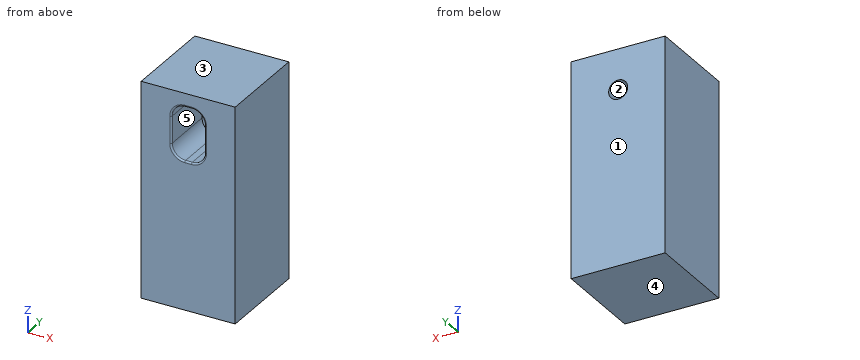
```python
from build123d import *

# Parameters (mm, degrees)
SKETCH1_W             = 22.225
SKETCH1_H             = 22.225
BOSS_EXTRUDE1_DEPTH   = 50.8
CUT_EXTRUDE1_DEPTH    = 12.7
F_8_CLEARANCE_HOLE1_D = 4.4958
FILLET1_R             = 0.381


with BuildPart() as part:
    # Sketch1 → Boss-Extrude1 (new body)
    with BuildSketch(Plane.XY):
        Rectangle(SKETCH1_W, SKETCH1_H)
    extrude(amount=BOSS_EXTRUDE1_DEPTH)

    # Sketch2 → Cut-Extrude1 (cut)
    with BuildSketch(Plane.XZ.offset(11.1125)):
        with BuildLine():
            Line((-0.79375, 47.625), (0.79375, 47.625))
            ThreePointArc((0.79375, 47.625), (3.03881403, 46.69506403), (3.96875, 44.45))
            Line((3.96875, 44.45), (3.96875, 38.1))
            ThreePointArc((3.96875, 38.1), (3.03881403, 35.85493597), (0.79375, 34.925))
            Line((0.79375, 34.925), (-0.79375, 34.925))
            ThreePointArc((-0.79375, 34.925), (-3.03881403, 35.85493597), (-3.96875, 38.1))
            Line((-3.96875, 38.1), (-3.96875, 44.45))
            ThreePointArc((-3.96875, 44.45), (-3.03881403, 46.69506403), (-0.79375, 47.625))
        make_face()
    extrude(amount=-CUT_EXTRUDE1_DEPTH, mode=Mode.SUBTRACT)

    # #8 Clearance Hole1 (through all)
    with Locations(Plane(origin=(0, 1.5875, 0), x_dir=(-1, 0, 0), z_dir=(0, -1, 0))):
        with Locations((0, -41.275)):
            Hole(F_8_CLEARANCE_HOLE1_D / 2)

    # Fillet1
    fillet1_edges = [part.edges().sort_by_distance(p)[0] for p in [
        (0, -11.1125, 47.625),
        (3.96875, -11.1125, 41.275),
        (-3.03881403, -11.1125, 46.69506403),
        (-3.96875, -11.1125, 41.275),
        (-3.03881403, -11.1125, 35.85493597),
        (0, -11.1125, 34.925),
        (3.03881403, -11.1125, 35.85493597),
        (3.03881403, -11.1125, 46.69506403),
    ]]
    fillet(fillet1_edges, radius=FILLET1_R)


solid = part.part
```
Design review of the part built by this model. Coordinates are the model's own, in mm. Face numbers are marked on the shaded views. A direction names the side the tool comes from. Give positions to 0.01 mm unless a question says otherwise; leave off trailing zeros. Order: outer loops, then holes, each group sorted by start corner. A loop starts at its lowest first (then second) coordinate and runs counter-clockwise, first axis right, second up. Notation, with made-up numbers: (10, -14.5) -> (53, -14.5) arc R25 cw to (53, 14.5) -> close; hole circle Ø4 at (68, 60.5). An arc over 180 degrees is marked (long way). Write each question's results on one line, items separated by ' | '. Start each with the question number.
Q1. Machinability: for the marked faces 4 and 5, which of the approach directions +Z, -Z, +X, -X, +Y, -Y give a long, thin tool a straight path to every point of the face, cutting with its end or side? Answer none if there is none.
Q2. Add section A-A on x = 0. Give the boundary of the cut face in (y, z) (1 decimal), and give its area (3 significant figures).
Q3. Wall thickness on L1, parallel to Z at x = 0, y = 8.25; L2, parallel to Z at x = -0.5, y = -7.5 (3 decimals); L3, parallel to Y at x = -3.5, z = 44: over which ranges is each line inside the solid? List them lowest first. Write a range as from..to.
Q4. Mouldability with a two-part tool opening along Z and no side actions: class the marked faces 1, 2 and 3 as +Z half, -Z half, draft (parallel to the pull), parting line (faces both ways), or undercut.
Q5. For pin 1 (2.5 mm diameter, centred on x = 0.5, z = 40, fed in from -Y), flat-tipped, find the tip position at first contact; note if it passes through.
Found:
1) face 4: -Z, +X, -X, +Y, -Y | face 5: -Y
2) outline: (-11.1, 0) -> (11.1, 0) -> (11.1, 39) -> (1.6, 39) -> (1.6, 34.9) -> (-10.7, 34.9) arc R0.4 ccw to (-11.1, 34.5) -> close; (-11.1, 48) arc R0.4 ccw to (-10.7, 47.6) -> (1.6, 47.6) -> (1.6, 43.5) -> (11.1, 43.5) -> (11.1, 50.8) -> (-11.1, 50.8) -> close | area: 925 mm2
3) L1: z = 0..39.03, 43.52..50.8 | L2: z = 0..34.925, 47.625..50.8 | L3: y = 1.59..11.11
4) face 1: draft | face 2: undercut | face 3: +Z half
5) pin 1: stops at y = 1.59
